Build history of the part. All positions in model axes, mm. A direction names the side the tool comes from. Round coordinates to 2 decimals unless told otherwise and drop trailing zeros. Write each loop counter-clockwise with the first axis right and the second up, starting at its lowest first coordinate (ties: lowest second). Pieces come first, ordered by that corner, then holes. Notation, with made-up numbers: M 69.5,38.5 L 96.5,38.5 A35 cw 96.5,72.5 Z; hole C 84,38 d8. An arc over 180 degrees is marked long. Write item = value, one per line.
from build123d import *

# Parameters (mm, degrees)
SKETCH1_R           = 1
BOSS_EXTRUDE1_DEPTH = 5


with BuildPart() as part:
    # Sketch1 → Boss-Extrude1 (new, symmetric)
    with BuildSketch(Plane.XY):
        Polygon((-20, 0), (20, 0), (20, 11), (15, 11), (10.050252532, 6.050252532), (10.050252532, 5.050252532), (-10.050252532, 5.050252532), (-10.050252532, 6.050252532), (-15, 11), (-20, 11), align=None)
        with Locations((-15, 6)):
            Circle(SKETCH1_R, mode=Mode.SUBTRACT)
        with Locations(Location((15, 6, 0), (0, 0, 180))):
            Circle(SKETCH1_R, mode=Mode.SUBTRACT)
    extrude(amount=BOSS_EXTRUDE1_DEPTH, both=True)


solid = part.part
1. Flat gauge pins, fed straight in: pin 1 (1.5 mm diameter, centred on x = -6, z = -2.5, fed in from +Y); pin 2 (2 mm diameter, centred on x = 10, z = 3.5, fed in from +Y). Where does each tip first touch, or does it go through?
Responses:
pin_1 = 5.05
pin_2 = 7
2. Band-saw the part on C-C (x = 0). List the corners of the cut face in (y, z), plus the area to 3 significant figures.
Responses:
outline = M 0,-5 L 5.05,-5 L 5.05,5 L 0,5 Z
area = 50.5 mm²
3. Tool access for faces 1 (the face through (13, 9, 0)), 2 (the face through (-17, 11, 0)): list every direction of +Z, -Z, +X, -X, +Y, -Y with a clear straight run to the whole face (end or side of a thin tool).
Responses:
face_1 = +Z, -Z, +Y
face_2 = +Z, -Z, +X, -X, +Y
4. Band-saw the part on D-D (x = -12). List the corners of the cut face in (y, z).
Responses:
outline = M 0,-5 L 8,-5 L 8,5 L 0,5 Z
5. Band-saw the part on B-B (z = -0.25). List the corners of the cut face in (x, y), plus the area to 3 significant figures.
Responses:
outline = M -20,0 L 20,0 L 20,11 L 15,11 L 10.05,6.05 L 10.05,5.05 L -10.05,5.05 L -10.05,6.05 L -15,11 L -20,11 Z; hole C -15,6 d2; hole C 15,6 d2
area = 290 mm²
6. Mould opens along Y. For faces 3 (the face through (20, 5, 0)), 4 (the face through (-14, 6, 0)), 5 (the face through (0, 5.05, 0)) say: pulls with the +Y half, pulls with the -Y half, needs draft (parallel to the pull), parting line crosses it, or undercut.
Responses:
face_3 = needs draft
face_4 = undercut
face_5 = pulls with the +Y half
7. Band-saw the part on A-A (y = 7.75). List the corners of the cut face in (x, z), plus the area to 3 significant figures.
Responses:
outline = M -20,-5 L -11.75,-5 L -11.75,5 L -20,5 Z; M 11.75,-5 L 20,-5 L 20,5 L 11.75,5 Z
area = 165 mm²
8. Probe probe 1 along Y at (x, z) = (-2, -2.25); probe 2 along Y at (x, z) = (15, -2.75); probe 3 along Y at (x, z) = (-15.5, -0.75). List the from-to ranges inside material, lowest first.
Responses:
probe_1 = 0 to 5.05
probe_2 = 0 to 5, 7 to 11
probe_3 = 0 to 5.13, 6.87 to 11
